The listing builds one solid part. Answer for the finished solid, in the listing's coordinates (mm). A direction names the side the tool comes from. Give positions to 0.01 mm unless a question says otherwise; leave off trailing zeros. Order: outer loops, then holes, each group sorted by start corner. A loop starts at its lowest first (then second) coordinate and runs counter-clockwise, first axis right, second up. Notation, with made-up numbers: (19.25, -16.5) - (49.25, -16.5) arc R15 cw to (49.25, -6.5) - close; hole circle Ø2 at (42, 23). An arc over 180 degrees is marked (long way). Answer as CSV lines item,"result". Start each with the question number.
1. Section A-A on x = 25.4 is taken. Give the vertices of the cut face in (y, z) (1 decimal).
2. Consider line 1 along Y through (x, z) = (25.4, 0.8); line 2 along Y through (x, z) = (8.5, 47) (3 decimals); line 3 along Z through (x, y) = (40, -24) (3 decimals). Determine where each line is inside the solid, lowest interval first. Write a range as [from, to].
3. Section B-B on y = -23 is taken. Give the vertices of the cut face in (x, z) (3 decimals).
4. Which of the six approach directions +Z, -Z, +X, -X, +Y, -Y give full straight-line access (tool end or side, diameter ignored) to faces 1 (the flat face through (25, -3.175, 27)), 2 (the flat face through (0, -14, 3))?
5. Section D-D on y = -35.5 is taken. Give the vertices of the cut face in (x, z) (3 decimals), and give its area (3 significant figures).
6. Flat-ended cylindrical pins translate along their axes: pin 1 (1 mm diameter, centred on x = 5, z = 28, fed in from -Y) (3 decimals); pin 2 (10 mm diameter, centred on x = 17, y = -42.5, fed in from +Z) (3 decimals); pin 3 (5 mm diameter, centred on x = 27, z = 19, fed in from +Y). Find the tip coordinate at first contact, or state that the pin passes through.
7. Determine the mould class of faces 3 (the flat face through (50.8, -14, 3)), 4 (the cylindrical face through (24.023, -33.186, 1.61)), 5 (the flat face through (31, -32, 3.175)) for opening direction X: +X half, -X half, draft (parallel to the pull), parting line (faces both ways), or undercut.
8. Section C-C on z = 18 is taken. Give the vertices of the cut face in (x, y) (3 decimals).
from build123d import *

# Parameters (mm, degrees)
F1_DEPTH = 50.8
F2_R     = 6.35
F3_DEPTH = 25.4


with BuildPart() as f1:
    # F0 (on Right) → F1 (new body)
    with BuildSketch(Plane.YZ):
        Polygon((-50.8, 0), (0, 0), (0, 50.8), (-3.175, 50.8), (-3.175, 3.175), (-50.8, 3.175), align=None)
    extrude(amount=F1_DEPTH)

    # F2 (on face) → F3 (cut)
    with BuildSketch(Plane.XY.offset(3.175)):
        with Locations((25.4, -26.9875)):
            Circle(F2_R)
    extrude(amount=-F3_DEPTH, mode=Mode.SUBTRACT)


solid = f1.part
Checks:
1,outline,"(-50.8, 0) - (-33.3, 0) - (-33.3, 3.2) - (-50.8, 3.2) - close; (-20.6, 0) - (0, 0) - (0, 50.8) - (-3.2, 50.8) - (-3.2, 3.2) - (-20.6, 3.2) - close"
2,line 1,"y = [-50.8, -33.34], [-20.64, 0]"
2,line 2,"y = [-3.175, 0]"
2,line 3,"z = [0, 3.175]"
3,outline,"(0, 0) - (20.458, 0) - (20.458, 3.175) - (0, 3.175) - close; (30.342, 0) - (50.8, 0) - (50.8, 3.175) - (30.342, 3.175) - close"
4,face 1,"+Z, +X, -X, -Y"
4,face 2,"+Z, -Z, -X, +Y, -Y"
5,outline,"(0, 0) - (50.8, 0) - (50.8, 3.175) - (0, 3.175) - close"
5,area,"161 mm²"
6,pin 1,"stops at y = -3.175"
6,pin 2,"stops at z = 3.175"
6,pin 3,"stops at y = 0"
7,face 3,"+X half"
7,face 4,"undercut"
7,face 5,"draft"
8,outline,"(0, -3.175) - (50.8, -3.175) - (50.8, 0) - (0, 0) - close"
